Solid Edge part; units mm, degrees
sketch "Sketch1" plane through (0, 0, 0) normal (0, -1, 0) x (1, 0, 0)
  line L0 (-12, -6) -> (12, -6)
  line L1 (12, -6) -> (12, 6)
  line L2 (12, 6) -> (-12, 6)
  line L3 (-12, 6) -> (-12, -6)
  line L4 (-15, -9) -> (15, -9)
  line L5 (15, -9) -> (15, 9)
  line L6 (15, 9) -> (-15, 9)
  line L7 (-15, 9) -> (-15, -9)
  dimension "D1" = 12
  dimension "D2" = 12
extrude "body" add sketch "Sketch1" against normal blind 10
sketch "Sketch2" plane through (0, 10, 0) normal (0, 1, 0) x (0, 0, -1)
  line L0 (-9, 11.5519) -> (-6, 3.3095)
  line L1 (-6, 3.3095) -> (-6, -4)
  line L2 (-6, -4) -> (-9, 4.2424)
  line L3 (-9, 4.2424) -> (-9, 11.5519)
  dimension "D1" = 6
extrude "Cutout1" cut sketch "Sketch2" against normal through all
properties material "Polyethylene, low density"
Verification items for the finished model (mm, model axes). A direction names the side the tool comes from. Give positions to 0.01 mm unless a question says otherwise; leave off trailing zeros. Order: outer loops, then holes, each group sorted by start corner. A loop starts at its lowest first (then second) coordinate and runs counter-clockwise, first axis right, second up. Notation, with made-up numbers: (-21.75, 5) -> (18.25, 5) arc R16 ccw to (18.25, 31) -> close; hole circle Ø2 at (63, 70.25). An arc over 180 degrees is marked (long way). Answer as CSV lines item,"result".
Q1. Scan lines: probe 1 along X at (y, z) = (1.25, 3.25); probe 2 along Z at (x, y) = (11.25, 3); probe 3 along Z at (x, y) = (-1.5, 5.5). Record each from-to range of solid material in increasing order.
Solutions:
probe 1,"x = -15 to -12, 12 to 15"
probe 2,"z = -9 to -6, 6 to 9"
probe 3,"z = -9 to -6, 8 to 9"
Q2. Sectioned sample at C-C on y = 6.75. Record the cut outline in (x, z).
Solutions:
outline,"(-15, -9) -> (15, -9) -> (15, 9) -> (-4.24, 9) -> (4, 6) -> (12, 6) -> (12, -6) -> (-12, -6) -> (-12, 6) -> (-3.31, 6) -> (-11.55, 9) -> (-15, 9) -> close"
Q3. Access from +Z, -Z, +X, -X, +Y, -Y to the whole of each face (thin tool, end or side, straight path). Record for faces 4 (the flat face through (-8, 5, 6)), 5 (the flat face through (0, 0, 8)).
Solutions:
face 4,"+Y, -Y"
face 5,"+Z, -Z, +X, -X, -Y"
Q4. Sectioned sample at B-B on z = -2.75. Record the cut outline in (x, y), plus the area to 3 significant figures.
Solutions:
outline,"(-15, 0) -> (-12, 0) -> (-12, 10) -> (-15, 10) -> close; (12, 0) -> (15, 0) -> (15, 10) -> (12, 10) -> close"
area,"60.0 mm²"
Q5. Sectioned sample at A-A on x = 7.5. Record the cut outline in (y, z), plus the area to 3 significant figures.
Solutions:
outline,"(0, -9) -> (10, -9) -> (10, -6) -> (0, -6) -> close; (0, 6) -> (10, 6) -> (10, 9) -> (0, 9) -> close"
area,"60.0 mm²"
Q6. Release check for a two-part mould opening along Z. For faces 1 (the flat face through (-15, 5, 0)), 2 (the flat face through (0, 5, -9)), 3 (the flat face through (8, 5, 6)) record: +Z half, -Z half, draft (parallel to the pull), parting line (faces both ways), or undercut.
Solutions:
face 1,"draft"
face 2,"-Z half"
face 3,"undercut"
